from build123d import *

# Parameters (mm, degrees)
MAIN_SHAPE_PROFILE_W          = 57.15
MAIN_SHAPE_PROFILE_H          = 6.35
O_RINGS_PROFILE_W             = 2.032
O_RINGS_PROFILE_H             = 2.032
INJECTOR_WELL_PROFILE_R       = 6.35
INJECTOR_WELL_DEPTH           = 2.54
DOWEL_HOLES_PROFILE_R         = 1.27
DOWEL_HOLES_DEPTH             = 2.54
INJECTOR_HOLES_R              = 0.7493
CIRCULAR_INJECTOR_HOLES_DEPTH = 81.912057816


with BuildPart() as part:
    # Main Shape Profile → Main Shape (revolve)
    with BuildSketch(Plane.XY, mode=Mode.PRIVATE) as main_shape_sk:
        with Locations((28.575, 3.175)):
            Rectangle(MAIN_SHAPE_PROFILE_W, MAIN_SHAPE_PROFILE_H)
    revolve(main_shape_sk.sketch.rotate(Axis((0, 0, 0), (0, -1, 0)), 180), axis=Axis((0, 0, 0), (0, -1, 0)))

    # O Rings Profile → O-Rings Cutout (revolve, cut)
    with BuildSketch(Plane.XY, mode=Mode.PRIVATE) as o_rings_cutout_sk:
        with Locations((53.594, 5.334)):
            Rectangle(O_RINGS_PROFILE_W, O_RINGS_PROFILE_H)
        with Locations((53.594, 1.016)):
            Rectangle(O_RINGS_PROFILE_W, O_RINGS_PROFILE_H)
    revolve(o_rings_cutout_sk.sketch.rotate(Axis((0, 0, 0), (0, -1, 0)), 90), axis=Axis((0, 0, 0), (0, -1, 0)), mode=Mode.SUBTRACT)

    # Injector Well Profile → Injector Well (cut)
    with BuildSketch(Plane(origin=(0, 6.35, 0), x_dir=(1, 0, 0), z_dir=(0, 1, 0))):
        with BuildLine():
            Line((-38.1, 8.57504), (-20.504129194, 8.57504))
            ThreePointArc((-20.504129194, 8.57504), (0, 22.225), (20.504129194, 8.57504))
            Line((20.504129194, 8.57504), (38.1, 8.57504))
            ThreePointArc((38.1, 8.57504), (46.67504, 0), (38.1, -8.57504))
            Line((38.1, -8.57504), (20.504129194, -8.57504))
            ThreePointArc((20.504129194, -8.57504), (0, -22.225), (-20.504129194, -8.57504))
            Line((-20.504129194, -8.57504), (-38.1, -8.57504))
            ThreePointArc((-38.1, -8.57504), (-46.67504, 0), (-38.1, 8.57504))
        make_face()
        with Locations(Location((0, 0, 0), (0, 0, 180))):
            Circle(INJECTOR_WELL_PROFILE_R, mode=Mode.SUBTRACT)
    extrude(amount=-INJECTOR_WELL_DEPTH, mode=Mode.SUBTRACT)

    # Dowel Holes Profile → Dowel Holes (cut)
    with BuildSketch(Plane(origin=(0, 6.35, 0), x_dir=(1, 0, 0), z_dir=(0, 1, 0))):
        with Locations(Location((0, 25.4, 0), (0, 0, 180))):
            Circle(DOWEL_HOLES_PROFILE_R)
        with Locations(Location((0, 46.355, 0), (0, 0, 180))):
            Circle(DOWEL_HOLES_PROFILE_R)
        with Locations(Location((0, -46.355, 0), (0, 0, 180))):
            Circle(DOWEL_HOLES_PROFILE_R)
        with Locations(Location((0, -25.4, 0), (0, 0, 180))):
            Circle(DOWEL_HOLES_PROFILE_R)
    extrude(amount=-DOWEL_HOLES_DEPTH, mode=Mode.SUBTRACT)

    # Injector Holes → Circular Injector Holes (cut, through all)
    with BuildSketch(Plane(origin=(0, 3.81, 0), x_dir=(1, 0, 0), z_dir=(0, 1, 0))):
        with Locations(Location((0, -17.78, 0), (0, 0, 180))):
            Circle(INJECTOR_HOLES_R)
        with Locations(Location((0, -13.97, 0), (0, 0, 180))):
            Circle(INJECTOR_HOLES_R)
        with Locations(Location((0, -10.16, 0), (0, 0, 180))):
            Circle(INJECTOR_HOLES_R)
        with Locations(Location((-6.081118148, -16.707734798, 0), (0, 0, 180))):
            Circle(INJECTOR_HOLES_R)
        with Locations(Location((-11.4287637, -13.620270199, 0), (0, 0, 180))):
            Circle(INJECTOR_HOLES_R)
        with Locations(Location((-15.397931679, -8.89, 0), (0, 0, 180))):
            Circle(INJECTOR_HOLES_R)
        with Locations(Location((-17.509881849, -3.087464599, 0), (0, 0, 180))):
            Circle(INJECTOR_HOLES_R)
        with Locations(Location((-17.509881849, 3.087464599, 0), (0, 0, 180))):
            Circle(INJECTOR_HOLES_R)
        with Locations(Location((-15.397931679, 8.89, 0), (0, 0, 180))):
            Circle(INJECTOR_HOLES_R)
        with Locations(Location((-11.4287637, 13.620270199, 0), (0, 0, 180))):
            Circle(INJECTOR_HOLES_R)
        with Locations(Location((-6.081118148, 16.707734798, 0), (0, 0, 180))):
            Circle(INJECTOR_HOLES_R)
        with Locations(Location((0, 17.78, 0), (0, 0, 180))):
            Circle(INJECTOR_HOLES_R)
        with Locations(Location((6.081118148, 16.707734798, 0), (0, 0, 180))):
            Circle(INJECTOR_HOLES_R)
        with Locations(Location((11.4287637, 13.620270199, 0), (0, 0, 180))):
            Circle(INJECTOR_HOLES_R)
        with Locations(Location((15.397931679, 8.89, 0), (0, 0, 180))):
            Circle(INJECTOR_HOLES_R)
        with Locations(Location((17.509881849, 3.087464599, 0), (0, 0, 180))):
            Circle(INJECTOR_HOLES_R)
        with Locations(Location((17.509881849, -3.087464599, 0), (0, 0, 180))):
            Circle(INJECTOR_HOLES_R)
        with Locations(Location((15.397931679, -8.89, 0), (0, 0, 180))):
            Circle(INJECTOR_HOLES_R)
        with Locations(Location((11.4287637, -13.620270199, 0), (0, 0, 180))):
            Circle(INJECTOR_HOLES_R)
        with Locations(Location((-6.061355835, -12.586535085, 0), (0, 0, 180))):
            Circle(INJECTOR_HOLES_R)
        with Locations(Location((-10.92218581, -8.710152532, 0), (0, 0, 180))):
            Circle(INJECTOR_HOLES_R)
        with Locations(Location((-13.619742933, -3.108617447, 0), (0, 0, 180))):
            Circle(INJECTOR_HOLES_R)
        with Locations(Location((-13.619742933, 3.108617447, 0), (0, 0, 180))):
            Circle(INJECTOR_HOLES_R)
        with Locations(Location((-10.92218581, 8.710152532, 0), (0, 0, 180))):
            Circle(INJECTOR_HOLES_R)
        with Locations(Location((-6.061355835, 12.586535085, 0), (0, 0, 180))):
            Circle(INJECTOR_HOLES_R)
        with Locations(Location((0, 13.97, 0), (0, 0, 180))):
            Circle(INJECTOR_HOLES_R)
        with Locations(Location((6.061355835, 12.586535085, 0), (0, 0, 180))):
            Circle(INJECTOR_HOLES_R)
        with Locations(Location((10.92218581, 8.710152532, 0), (0, 0, 180))):
            Circle(INJECTOR_HOLES_R)
        with Locations(Location((13.619742933, 3.108617447, 0), (0, 0, 180))):
            Circle(INJECTOR_HOLES_R)
        with Locations(Location((13.619742933, -3.108617447, 0), (0, 0, 180))):
            Circle(INJECTOR_HOLES_R)
        with Locations(Location((10.92218581, -8.710152532, 0), (0, 0, 180))):
            Circle(INJECTOR_HOLES_R)
        with Locations(Location((-5.971898163, -8.219612663, 0), (0, 0, 180))):
            Circle(INJECTOR_HOLES_R)
        with Locations(Location((-9.662734206, -3.139612663, 0), (0, 0, 180))):
            Circle(INJECTOR_HOLES_R)
        with Locations(Location((-9.662734206, 3.139612663, 0), (0, 0, 180))):
            Circle(INJECTOR_HOLES_R)
        with Locations(Location((-5.971898163, 8.219612663, 0), (0, 0, 180))):
            Circle(INJECTOR_HOLES_R)
        with Locations(Location((0, 10.16, 0), (0, 0, 180))):
            Circle(INJECTOR_HOLES_R)
        with Locations(Location((5.971898163, 8.219612663, 0), (0, 0, 180))):
            Circle(INJECTOR_HOLES_R)
        with Locations(Location((9.662734206, 3.139612663, 0), (0, 0, 180))):
            Circle(INJECTOR_HOLES_R)
        with Locations(Location((9.662734206, -3.139612663, 0), (0, 0, 180))):
            Circle(INJECTOR_HOLES_R)
        with Locations(Location((5.971898163, -8.219612663, 0), (0, 0, 180))):
            Circle(INJECTOR_HOLES_R)
        with Locations(Location((6.061355835, -12.586535085, 0), (0, 0, 180))):
            Circle(INJECTOR_HOLES_R)
        with Locations(Location((6.081118148, -16.707734798, 0), (0, 0, 180))):
            Circle(INJECTOR_HOLES_R)
    extrude(amount=-CIRCULAR_INJECTOR_HOLES_DEPTH, mode=Mode.SUBTRACT)


solid = part.part
The model under review builds one solid part; all positions refer to its coordinate system, in mm. A direction names the side the tool comes from. Round coordinates to 2 decimals unless told otherwise and drop trailing zeros. Loops run counter-clockwise (first coordinate to the right, second up) from the corner with the lowest first, then second, coordinate; pieces in that order, holes last. Notation, with made-up numbers: M -26,-5.75 L 27,-5.75 A17 cw 27,20.25 Z; hole C 70.25,43 d10. An arc over 180 degrees is marked long. Answer as CSV lines item,"result".
1. To check wall thickness, follow L1, parallel to X at y = 5.5, z = 14; L2, parallel to X at y = 4.75, z = 41; L3, parallel to Z at x = -9.5, y = 5. State the ranges of each line that lie inside material, in increasing order. Write a range as [from, to].
Outcome:
L1,"x = [-55.41, -52.78], [-50.68, -17.26], [17.26, 50.68], [52.78, 55.41]"
L2,"x = [-39.81, -36.07], [-32.92, 32.92], [36.07, 39.81]"
L3,"z = [-56.35, -53.78], [-51.71, -20.09], [20.09, 51.71], [53.78, 56.35]"
2. We need section C-C (z = -40). Give the boundary of the cut face in (x, y), plus the area to 3 significant figures.
Outcome:
outline,"M -40.82,0 L -37.18,0 L -37.18,2.03 L -34.12,2.03 L -34.12,0 L 34.12,0 L 34.12,2.03 L 37.18,2.03 L 37.18,0 L 40.82,0 L 40.82,6.35 L 37.18,6.35 L 37.18,4.32 L 34.12,4.32 L 34.12,6.35 L -34.12,6.35 L -34.12,4.32 L -37.18,4.32 L -37.18,6.35 L -40.82,6.35 Z"
area,"494 mm2"
3. We need section B-B (x = -48.5). Give the boundary of the cut face in (y, z), plus the area to 3 significant figures.
Outcome:
outline,"M 0,-30.23 L 6.35,-30.23 L 6.35,-25.1 L 4.32,-25.1 L 4.32,-20.3 L 6.35,-20.3 L 6.35,20.3 L 4.32,20.3 L 4.32,25.1 L 6.35,25.1 L 6.35,30.23 L 0,30.23 L 0,25.1 L 2.03,25.1 L 2.03,20.3 L 0,20.3 L 0,-20.3 L 2.03,-20.3 L 2.03,-25.1 L 0,-25.1 Z"
area,"345 mm2"
4. We need section A-A (z = 0). Give the boundary of the cut face in (x, y).
Outcome:
outline,"M -57.15,0 L -54.61,0 L -54.61,2.03 L -52.58,2.03 L -52.58,0 L 52.58,0 L 52.58,2.03 L 54.61,2.03 L 54.61,0 L 57.15,0 L 57.15,6.35 L 54.61,6.35 L 54.61,4.32 L 52.58,4.32 L 52.58,6.35 L 46.68,6.35 L 46.68,3.81 L 6.35,3.81 L 6.35,6.35 L -6.35,6.35 L -6.35,3.81 L -46.68,3.81 L -46.68,6.35 L -52.58,6.35 L -52.58,4.32 L -54.61,4.32 L -54.61,6.35 L -57.15,6.35 Z"
5. Insertion check: pin 1 Ø4 at (x, z) = (9, -16) entering from +Y; pin 2 Ø1.5 at (y, z) = (4, -13.5) entering from +X; pin 3 Ø1.5 at (x, y) = (24.5, 5) entering from +Z. Each pin has a flat end and moves straight along its axis. Give the tip position at first contact, or say it passes through.
Outcome:
pin 1,"stops at y = 3.81"
pin 2,"stops at x = 55.71"
pin 3,"stops at z = 51.98"
6. We need section D-D (x = -30.5). Give the boundary of the cut face in (y, z).
Outcome:
outline,"M 0,-48.33 L 6.35,-48.33 L 6.35,-45.3 L 4.32,-45.3 L 4.32,-42.83 L 6.35,-42.83 L 6.35,-8.58 L 3.81,-8.58 L 3.81,8.58 L 6.35,8.58 L 6.35,42.83 L 4.32,42.83 L 4.32,45.3 L 6.35,45.3 L 6.35,48.33 L 0,48.33 L 0,45.3 L 2.03,45.3 L 2.03,42.83 L 0,42.83 L 0,-42.83 L 2.03,-42.83 L 2.03,-45.3 L 0,-45.3 Z"
7. For faces 4 (the face through (-45, 4.318, 29)), 5 (the face through (-45, 2.032, 29)), list the 3-axis set-ups (+Z, -Z, +X, -X, +Y, -Y) from which the entire face can be reached by the end or side of a thin tool; tool diameter is ignored.
Outcome:
face 4,"+Y"
face 5,"-Y"
8. Draft analysis for pull direction Z (two halves, no side actions). For faces 1 (the face through (57.095, 3.219, -2.513)), 2 (the face through (0.28, 5.1, 24.16)), 3 (the face through (29.4, 6.35, 46.3)), state which applies: pulls with the +Z half, pulls with the -Z half, needs draft (parallel to the pull), parting line crosses it, or undercut.
Outcome:
face 1,"parting line crosses it"
face 2,"undercut"
face 3,"needs draft"
